from build123d import *

# Parameters (mm, degrees)
BOSS_EXTRUDE2_DEPTH = 25
CUT_EXTRUDE2_REACH  = 149.893
SKETCH4_R           = 2
SKETCH4_R_2         = 4
CUT_EXTRUDE3_REACH  = 146.42
SKETCH5_R           = 2.5


with BuildPart() as part:
    # Sketch3 → Boss-Extrude2 (new, symmetric)
    with BuildSketch(Plane(origin=(0, 0, 0), x_dir=(1, 0, 0), z_dir=(0, 1, 0))):
        Polygon((0, 0), (5, 0), (5, 136.5), (40, 136.5), (40, 141.5), (0, 141.5), align=None)
    extrude(amount=BOSS_EXTRUDE2_DEPTH, both=True)

    # Sketch4 → Cut-Extrude2 (cut, up to next)
    with BuildSketch(Plane(origin=(5, 0, 0), x_dir=(0, 0, -1), z_dir=(1, 0, 0)), mode=Mode.PRIVATE) as cut_extrude2_sk1:
        with Locations((4, 15.5)):
            Circle(SKETCH4_R)
    cut_extrude2_tool1 = extrude(cut_extrude2_sk1.sketch, amount=-CUT_EXTRUDE2_REACH, mode=Mode.PRIVATE) & part.part
    # Sketch4 → Cut-Extrude2 (cut, up to next)
    with BuildSketch(Plane(origin=(5, 0, 0), x_dir=(0, 0, -1), z_dir=(1, 0, 0)), mode=Mode.PRIVATE) as cut_extrude2_sk2:
        with Locations((29, 15.5)):
            Circle(SKETCH4_R_2)
    cut_extrude2_tool2 = extrude(cut_extrude2_sk2.sketch, amount=-CUT_EXTRUDE2_REACH, mode=Mode.PRIVATE) & part.part
    add(cut_extrude2_tool1.solids().sort_by_distance((5, 15.5, -4))[0], mode=Mode.SUBTRACT)
    add(cut_extrude2_tool2.solids().sort_by_distance((5, 15.5, -29))[0], mode=Mode.SUBTRACT)

    # Sketch5 → Cut-Extrude3 (cut, up to next)
    with BuildSketch(Plane.XY.offset(-136.5), mode=Mode.PRIVATE) as cut_extrude3_sk1:
        with Locations((22.5, 12.5)):
            Circle(SKETCH5_R)
    cut_extrude3_tool1 = extrude(cut_extrude3_sk1.sketch, amount=-CUT_EXTRUDE3_REACH, mode=Mode.PRIVATE) & part.part
    # Sketch5 → Cut-Extrude3 (cut, up to next)
    with BuildSketch(Plane.XY.offset(-136.5), mode=Mode.PRIVATE) as cut_extrude3_sk2:
        with Locations((22.5, -12.5)):
            Circle(SKETCH5_R)
    cut_extrude3_tool2 = extrude(cut_extrude3_sk2.sketch, amount=-CUT_EXTRUDE3_REACH, mode=Mode.PRIVATE) & part.part
    add(cut_extrude3_tool1.solids().sort_by_distance((22.5, 12.5, -136.5))[0], mode=Mode.SUBTRACT)
    add(cut_extrude3_tool2.solids().sort_by_distance((22.5, -12.5, -136.5))[0], mode=Mode.SUBTRACT)


solid = part.part
Geometry check sheet. Reference: the model listing, model coordinates, mm. Give positions to 0.01 mm unless a question says otherwise; leave off trailing zeros. Order: outer loops, then holes, each group sorted by start corner. A loop starts at its lowest first (then second) coordinate and runs counter-clockwise, first axis right, second up.
1) Cross-section at B-B (y = -12.5). Record the boundary of the cut face in (x, z).
Results are:
outline: (0, -141.5) - (20, -141.5) - (20, -136.5) - (5, -136.5) - (5, 0) - (0, 0) - close; (25, -141.5) - (40, -141.5) - (40, -136.5) - (25, -136.5) - close
2) Material ranges on probe 1 along Y at (x, z) = (22.5, -138.85); probe 2 along Y at (x, z) = (1.75, -29); probe 3 along Y at (x, z) = (2.65, -4), recorded low to high.
Results are:
probe 1: y = -25 to -15, -10 to 10, 15 to 25
probe 2: y = -25 to 11.5, 19.5 to 25
probe 3: y = -25 to 13.5, 17.5 to 25
3) Cross-section at A-A (z = -29). Record the boundary of the cut face in (x, y), then the cut area to 3 significant figures.
Results are:
outline: (0, -25) - (5, -25) - (5, 11.5) - (0, 11.5) - close; (0, 19.5) - (5, 19.5) - (5, 25) - (0, 25) - close
area: 210 mm2
4) Cross-section at D-D (y = -5). Record the boundary of the cut face in (x, z).
Results are:
outline: (0, -141.5) - (40, -141.5) - (40, -136.5) - (5, -136.5) - (5, 0) - (0, 0) - close
5) Draft check along X on faces 1 (the flat face through (22, 0, -136.5)), 2 (the cylindrical face through (20.5, -14, -139)), 3 (the flat face through (5, 0, -67)). Enter one of: released by +X, released by -X, zero draft, split by the parting line, or undercut.
Results are:
face 1: zero draft
face 2: undercut
face 3: released by +X
6) Gauge pin test, flat ends, axial feed: pin 1 (10.5 mm diameter, centred on x = 15, y = 7, fed in from +Z); pin 2 (9 mm diameter, centred on y = 15.5, z = -29, fed in from +X). Record the tip position at first contact, or that the pin passes through.
Results are:
pin 1: stops at z = -136.5
pin 2: stops at x = 5
7) Cross-section at C-C (x = 22.5). Record the boundary of the cut face in (y, z), then the cut area to 3 significant figures.
Results are:
outline: (-25, -141.5) - (-15, -141.5) - (-15, -136.5) - (-25, -136.5) - close; (-10, -141.5) - (10, -141.5) - (10, -136.5) - (-10, -136.5) - close; (15, -141.5) - (25, -141.5) - (25, -136.5) - (15, -136.5) - close
area: 200 mm2
